Input: part model. Units: mm. Frame: model coordinates. Face numbers are marked on the shaded views. Round coordinates to 2 decimals unless told otherwise and drop trailing zeros. One line per item, written item: value. Start each with the question number.
Autodesk Inventor part; units mm, degrees
ref_plane "YZ Plane" through (0, 0, 0) normal (1, 0, 0) x (0, 1, 0)
ref_plane "XZ Plane" through (0, 0, 0) normal (0, 1, 0) x (-1, 0, 0)
ref_plane "XY Plane" through (0, 0, 0) normal (0, 0, 1) x (1, 0, 0)
sketch "草圖1" plane through (0, 0, 0) normal (0, 1, 0) x (-1, 0, 0)
  line L0 (133, 0) -> (-133, 0) construction
  line L1 (0, -161) -> (0, 161) construction
  line L2 (95, -115) -> (-95, -115)
  line L3 (-95, -115) -> (-95, 115)
  line L4 (-95, 115) -> (95, 115)
  line L5 (95, 115) -> (95, -115)
  point P0 (0, 0)
  dimension "d0" = 190
  dimension "d1" = 230
extrude "擠出1" add sketch "草圖1" along normal blind 40
sketch "草圖3" plane through (0, 0, 0) normal (1, 0, 0) x (0, 1, 0)
  line L0 (0, 115) -> (0, -115) construction
  line L1 (0, 115) -> (40, 115) construction
  line L2 (40, -115) -> (40, 115) construction
  line L3 (0, -115) -> (40, -115) construction
  line L4 (-8, 0) -> (48, 0) construction
  line L5 (0, -161) -> (0, 161) construction
  line L6 (10, 107) -> (40, 107)
  line L7 (40, 107) -> (40, -107)
  line L8 (40, -107) -> (10, -107)
  line L9 (10, 107) -> (10, -107.0049)
  point P0 (0, 0)
  dimension "d13" = 8
  dimension "d14" = 8
  dimension "d27" = 10
sketch "草圖2" plane through (0, 40, 0) normal (0, 1, 0) x (1, 0, 0)
  line L0 (95, 115) -> (-95, 115) construction
  line L1 (-95, 115) -> (-95, -115) construction
  line L2 (-95, -115) -> (95, -115) construction
  line L3 (95, -115) -> (95, 115) construction
  line L4 (-133, 0) -> (133, 0) construction
  line L5 (0, 161) -> (0, -161) construction
  line L6 (-87, 107) -> (87, 107)
  line L7 (87, 107) -> (87, -107)
  line L8 (87, -107) -> (-87, -107)
  line L9 (-87, -107) -> (-87, 107)
  line L10 (-87, -80.0748) -> (45.1402, -87)
  line L11 (45.1402, -92) -> (-87, -92)
  line L12 (45.1402, -92) -> (45.1402, -87)
  line L13 (72, 53.3199) -> (72, -81.708)
  line L14 (72, -81.708) -> (67, -81.708)
  line L15 (67, -81.708) -> (67, 53.3199)
  arc A0 (67, 53.3199) -> (43.2398, 73.9691) centre (46.1471, 53.3199) ccw
  arc A1 (72, 53.3199) -> (42.5427, 78.9203) centre (46.1471, 53.3199) ccw
  line L16 (43.2398, 73.9691) -> (33.9304, 72.6584)
  line L17 (45.4216, 79.3256) -> (33.2333, 77.6096)
  line L18 (33.2333, 77.6096) -> (33.9304, 72.6584)
  point P0 (0, 0)
  dimension "d4" = 8
  dimension "d5" = 15
  dimension "d6" = 5
  dimension "d7" = 3
  dimension "d8" = 15
  dimension "d9" = 5
  dimension "d10" = 5
extrude "擠出7" cut sketch "草圖3" along normal mid plane 174
extrude "擠出8" add sketch "草圖2" against normal up to next contours L10 L12 L11 L9 | L13 L14 L15 A0 L16 L18 L17 A1
sketch "草圖6" plane through (-87, 10, 107) normal (0, 1, 0) x (1, 0, 0)
  line L0 (132.1402, 15) -> (0, 15)
  line L1 (0, 15) -> (0, 0)
  line L2 (0, 0) -> (174, 0)
  line L3 (174, 0) -> (174, 214)
  line L4 (0, 214) -> (174, 214)
  line L5 (0, 214) -> (0, 26.9252)
  line L6 (0, 26.9252) -> (132.1402, 20)
  line L7 (132.1402, 20) -> (132.1402, 15)
  arc A0 (159, 160.3199) -> (129.5427, 185.9203) centre (133.1471, 160.3199) ccw
  line L8 (159, 160.3199) -> (159, 25.292)
  line L9 (159, 25.292) -> (154, 25.292)
  line L10 (154, 25.292) -> (154, 160.3199)
  arc A1 (154, 160.3199) -> (130.2398, 180.9691) centre (133.1471, 160.3199) ccw
  line L11 (130.2398, 180.9691) -> (120.9304, 179.6584)
  line L12 (120.9304, 179.6584) -> (120.2333, 184.6096)
  line L13 (120.2333, 184.6096) -> (129.5427, 185.9203)
  point P0 (87, 107)
extrude "擠出9" add sketch "草圖6" along normal blind 15
sketch "草圖9" plane through (-95, 0, 115) normal (0, 0, 1) x (1, 0, 0)
  line L0 (182, 25) -> (8, 25) construction
  line L1 (182, 40) -> (182, 25) construction
  line L2 (167, 40) -> (167, 25) construction
  circle A0 centre (174.5, 32.5) radius 7.5
  point P0 (95, 0)
  dimension "d64" = 15
extrude "擠出11" cut sketch "草圖9" against normal blind 20
sketch "草圖10" plane through (0, 40, 0) normal (0, 1, 0) x (1, 0, 0)
  line L0 (-87, -92) -> (45.1402, -92) construction
  line L1 (45.1402, -92) -> (45.1402, -87) construction
  line L2 (45.1402, -87) -> (-87, -80.0748) construction
  line L3 (-87, -80.0748) -> (-87, 107)
  line L4 (-87, 107) -> (87, 107)
  line L5 (87, 107) -> (87, -107)
  line L6 (87, -107) -> (79.5, -107)
  line L7 (79.5, -115) -> (79.5, -107)
  line L8 (79.5, -115) -> (95, -115)
  line L9 (95, -115) -> (95, 115)
  line L10 (95, 115) -> (-95, 115)
  line L11 (-95, 115) -> (-95, -115)
  line L12 (-95, -115) -> (79.5, -115)
  line L13 (79.5, -107) -> (-87, -107)
  line L14 (-87, -107) -> (-87, -92)
  line L15 (-87, -80.0748) -> (-87, -92)
  point P0 (0, 0)
extrude "擠出12" add sketch "草圖10" along normal blind 5
fillet "圓角1" radius 50 1 edges at (87, 35, -107)
sketch "草圖11" plane through (-87, 25, 107) normal (0, 1, 0) x (1, 0, 0)
  line L0 (16.0333, 148.1759) -> (51.7064, 141.7244)
  line L1 (51.7064, 141.7244) -> (50.8968, 137.2481)
  line L2 (50.8968, 137.2481) -> (15.2237, 143.6996)
  line L3 (15.2237, 143.6996) -> (16.0333, 148.1759)
  line L4 (182, 222) -> (-8, 222)
  line L5 (70.9047, 222) -> (70.9047, 192.887) construction
  line L6 (125.7761, 148.1759) -> (90.103, 141.7244)
  line L7 (90.103, 141.7244) -> (90.9126, 137.2481)
  line L8 (90.9126, 137.2481) -> (126.5857, 143.6996)
  line L9 (126.5857, 143.6996) -> (125.7761, 148.1759)
  circle A0 centre (26.1565, 124.5773) radius 2.5
  circle A1 centre (11.4824, 101.8214) radius 2.5
  circle A2 centre (23.8526, 77.7353) radius 2.5
  circle A3 centre (50.8968, 76.4051) radius 2.5
  circle A4 centre (65.5709, 99.161) radius 2.5
  circle A5 centre (53.2008, 123.2471) radius 2.5
  circle A6 centre (126.3016, 41.8829) radius 2.5
  circle A7 centre (149.3019, 68.1668) radius 2.5
  circle A8 centre (143.0928, 102.5369) radius 2.5
  circle A9 centre (112.3498, 119.1118) radius 2.5
  circle A10 centre (80.2231, 105.4102) radius 2.5
  circle A11 centre (70.9047, 71.7498) radius 2.5
  circle A12 centre (91.4116, 43.4775) radius 2.5
  line L10 (95.0789, 88.3359) -> (132.687, 78.9051)
  line L11 (132.687, 78.9051) -> (131.5197, 74.2498)
  line L12 (131.5197, 74.2498) -> (93.9116, 83.6806)
  line L13 (93.9116, 83.6806) -> (95.0789, 88.3359)
  line L14 (38.5267, 40.9775) -> (73.475, 52.9247)
  line L15 (73.475, 52.9247) -> (74.6702, 49.4284)
  line L16 (74.6702, 49.4284) -> (39.7219, 37.4812)
  line L17 (39.7219, 37.4812) -> (38.5267, 40.9775)
  line L18 (12.2608, 69.2526) -> (39.4354, 58.057)
  line L19 (39.4354, 58.057) -> (37.5308, 53.434)
  line L20 (37.5308, 53.434) -> (10.3562, 64.6295)
  line L21 (10.3562, 64.6295) -> (12.2608, 69.2526)
  circle A13 centre (106.3327, 56.6592) radius 4
  circle A14 centre (123.8016, 102.7619) radius 4
  circle A15 centre (27.1857, 95.1306) radius 3.3162
  circle A16 centre (48.3968, 105.4102) radius 2.6483
  point P0 (38.5267, 100.4912)
  point P1 (110.5122, 78.9051)
  dimension "d70" = 5
  dimension "d73" = 360
  dimension "d75" = 5
  dimension "d78" = 360
  dimension "d80" = 5
  dimension "d81" = 8
  dimension "d82" = 8
extrude "擠出13" add sketch "草圖11" along normal up to surface (20 mm away)
properties part number "ball"
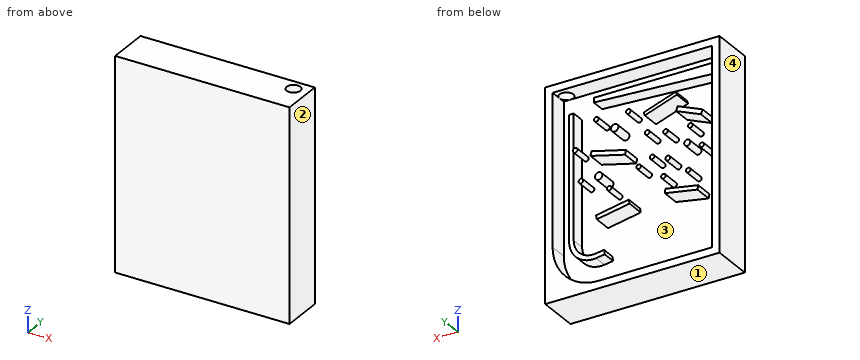
1. Pin query (flat end, axial travel): pin 1 (6 mm diameter, centred on x = -44.5, z = 85.5, fed in from +Y). Return the tip coordinate at first contact, or that it passes through.
2. Pull-direction query (X, two-part tool) for the marked faces 1, 2, 3 and 4; classes: released by +X, released by -X, zero draft, split by the parting line, or undercut.
3. Line query: line 1 (X direction, y = 32, z = -50.5); line 2 (X direction, y = 32.5, z = 112.25); line 3 (Y direction, x = 79.5, z = 113.25). Output: solid intervals per line, ascending. Write a range as from..to.
Solved:
1. pin 1: stops at y = 40
2. face 1: zero draft
2. face 2: released by +X
2. face 3: undercut
2. face 4: released by -X
3. line 1: x = -95..-87, 67..72, 87..95
3. line 2: x = -95..72, 87..95
3. line 3: y = 0..25, 40..45
